Autodesk Inventor part; units mm, degrees
ref_plane "YZ Plane" through (0, 0, 0) normal (1, 0, 0) x (0, 1, 0)
ref_plane "XZ Plane" through (0, 0, 0) normal (0, 1, 0) x (-1, 0, 0)
ref_plane "XY Plane" through (0, 0, 0) normal (0, 0, 1) x (1, 0, 0)
ref_plane "Work Plane1" through (-4.5, 4.3393, 236.083) normal (0, 0, -1) x (1, 0, 0)
sketch "Sketch1" plane through (-4.5, 4.3393, 236.083) normal (0, 0, -1) x (1, 0, 0)
  circle A0 centre (0, 4.1863) radius 17 construction
  line L0 (34.5, -9.3137) -> (34.5, 17.6863)
  line L1 (34.5, 17.6863) -> (25.5, 17.6863)
  line L2 (25.5, 17.6863) -> (25.5, 12.6863)
  line L3 (25.5, 12.6863) -> (30.5, 12.6863)
  line L4 (30.5, 12.6863) -> (30.5, -4.3137)
  line L5 (30.5, -4.3137) -> (25.5, -4.3137)
  line L6 (25.5, -4.3137) -> (25.5, -9.3137)
  line L7 (25.5, -9.3137) -> (34.5, -9.3137)
  line L8 (0, -8.3452) -> (0, -17.0863) construction
  line L9 (0, -12.8137) -> (-4, -12.8137)
  line L10 (-4, -12.8137) -> (-4, -16.8137)
  line L11 (-4, -16.8137) -> (30, -16.8137)
  line L12 (30, -16.8137) -> (38.5, -12.8501)
  line L13 (38.5, -12.8501) -> (38.5, 4.1863)
  arc A1 (0, -12.8137) -> (17, 4.1863) centre (0, 4.1863) ccw
  line L14 (0, 4.1863) -> (38.5, 4.1863) construction
  line L15 (0, 21.1863) -> (-4, 21.1863)
  line L16 (-4, 21.1863) -> (-4, 25.1863)
  line L17 (-4, 25.1863) -> (30, 25.1863)
  line L18 (30, 25.1863) -> (38.5, 21.2227)
  line L19 (38.5, 21.2227) -> (38.5, 4.1863)
  arc A2 (17, 4.1863) -> (0, 21.1863) centre (0, 4.1863) ccw
  point P0 (4.5, 4.3393)
  point P1 (0, 25.4589)
  dimension "d0" = 4
  dimension "d1" = 4
  dimension "d2" = 4
  dimension "d3" = 115
  dimension "d4" = 8.5
extrude "Extrusion1" add sketch "Sketch1" against normal blind 13
properties part number "giunto_fondo_siringa"
CAD build for the part. Positions are in the model's coordinates, mm. A direction names the side the tool comes from. Give positions to 0.01 mm unless a question says otherwise; leave off trailing zeros. Loops run counter-clockwise (first coordinate to the right, second up) from the corner with the lowest first, then second, coordinate; pieces in that order, holes last. Notation, with made-up numbers: M 10,-36 L 54,-36 A9 ccw 54,-29 Z; hole C 30.5,81 d5. An arc over 180 degrees is marked long. Answer in a Markdown table with one row per item. Add a question column.
Item 1: Band-saw the part on D-D on y = 16. Give the cut face in (x, z), then the cut area to 3 significant figures.
Item 2: Drop flat-ended pins along their axis: P1, Ø6.5, axis at y = 0, z = 240.5, coming from the -X side; P2, Ø2, axis at y = -1, z = 245, coming from the -X side. Give the stop position or say it passes through.
Item 3: Probe probe 1 along Y at (x, z) = (-4, 244); probe 2 along Y at (x, z) = (24, 245.75); probe 3 along Y at (x, z) = (-7, 245.25). List the from-to ranges inside material, lowest first.
Item 4: Tool access for faces 1 (the face through (-8.5, -19, 242)), 2 (the face through (-6, 17.153, 242)), 3 (the face through (24, 8.653, 242)): list every direction of +Z, -Z, +X, -X, +Y, -Y with a clear straight run to the whole face (end or side of a thin tool).
Item 5: Band-saw the part on B-B on y = 11.5. Give the cut face in (x, z), then the cut area to 3 significant figures.
Item 6: Band-saw the part on C-C on x = 8.5. Give the cut face in (y, z).
Item 7: Band-saw the part on A-A on z = 242. Give the cut face in (x, y), then the cut area to 3 significant figures.
Reply:
| question | item | result |
|---|---|---|
| 1 | outline | M 1.65,236.08 L 34,236.08 L 34,249.08 L 1.65,249.08 Z |
| 1 | area | 420 mm^2 |
| 2 | P1 | stops at x = 12.16 |
| 2 | P2 | stops at x = 12.36 |
| 3 | probe 1 | y = -20.85 to -16.84, 17.15 to 21.15 |
| 3 | probe 2 | y = -20.85 to -13.35, -8.35 to 8.65, 13.65 to 21.15 |
| 3 | probe 3 | y = -20.85 to -16.85, 17.15 to 21.15 |
| 4 | face 1 | +Z, -Z, -X, +Y, -Y |
| 4 | face 2 | +Z, -Z, -X |
| 4 | face 3 | +Z, -Z |
| 5 | outline | M 8.16,236.08 L 21,236.08 L 21,249.08 L 8.16,249.08 Z; M 30,236.08 L 34,236.08 L 34,249.08 L 30,249.08 Z |
| 5 | area | 219 mm^2 |
| 6 | outline | M -20.85,236.08 L -10.8,236.08 L -10.8,249.08 L -20.85,249.08 Z; M 11.11,236.08 L 21.15,236.08 L 21.15,249.08 L 11.11,249.08 Z |
| 7 | outline | M -8.5,-20.85 L 25.5,-20.85 L 34,-16.88 L 34,17.19 L 25.5,21.15 L -8.5,21.15 L -8.5,17.15 L -4.5,17.15 A17 cw -4.5,-16.85 L -8.5,-16.85 Z; hole M 21,-13.35 L 30,-13.35 L 30,13.65 L 21,13.65 L 21,8.65 L 26,8.65 L 26,-8.35 L 21,-8.35 Z |
| 7 | area | 1,000 mm^2 |
